Verification items for the finished model (mm, model axes). Round coordinates to 2 decimals unless told otherwise and drop trailing zeros. Write each loop counter-clockwise with the first axis right and the second up, starting at its lowest first coordinate (ties: lowest second). Pieces come first, ordered by that corner, then holes. Notation, with made-up numbers: M 0.25,43 L 30.25,43 A30 ccw 30.25,76 Z; hole C -24.5,-27 d4. An arc over 180 degrees is marked long. Answer in a Markdown table with one row per item. Add a question column.
1. Sectioned sample at C-C on y = -19.5. Record the cut outline in (x, z), plus the area to 3 significant figures.
2. Material ranges on probe 1 along Y at (x, z) = (52, 1563); probe 2 along X at (y, z) = (-2, 1149), recorded low to high.
3. Go/stop test with flat-tipped pins: pin 1 Ø1.5 at (y, z) = (-46.5, 614) entering from -X; pin 2 Ø10 at (y, z) = (-34, 258) entering from +X. Record where each tip stops, or that it passes through.
4. Sectioned sample at A-A on x = -25. Record the cut outline in (y, z), plus the area to 3 significant figures.
5. Sectioned sample at B-B on z = 566.5. Record the cut outline in (x, y), plus the area to 3 significant figures.
```python
from build123d import *

# Parameters (mm, degrees)
BOSS_EXTRUDE1_DEPTH = 2133.6
SKETCH2_W           = 19.05
SKETCH2_H           = 19.05
CUT_EXTRUDE1_DEPTH  = 2136.489044692
FILLET1_R           = 2.54


with BuildPart() as part:
    # Sketch1 → Boss-Extrude1 (new body)
    with BuildSketch(Plane.XY):
        Polygon((-63.5, 63.5), (63.5, 63.5), (63.5, 53.0352), (23.0251, 53.0352), (23.0251, 33.9852), (3.9751, 33.9852), (3.9751, -53.0352), (63.5, -53.0352), (63.5, -63.5), (-63.5, -63.5), (-63.5, -53.0352), (-3.9751, -53.0352), (-3.9751, 33.9852), (-23.0251, 33.9852), (-23.0251, 53.0352), (-63.5, 53.0352), align=None)
    extrude(amount=BOSS_EXTRUDE1_DEPTH)

    # Sketch2 → Cut-Extrude1 (cut, through all)
    with BuildSketch(Plane.XY):
        with Locations((-13.5001, 43.5102)):
            Rectangle(SKETCH2_W, SKETCH2_H)
        with Locations((13.5001, 43.5102)):
            Rectangle(SKETCH2_W, SKETCH2_H)
    extrude(amount=CUT_EXTRUDE1_DEPTH, mode=Mode.SUBTRACT)

    # Fillet1
    fillet1_edges = [part.edges().sort_by_distance(p)[0] for p in [
        (-63.5, -53.0352, 1066.8),
        (-3.9751, -53.0352, 1066.8),
        (-63.5, 53.0352, 1066.8),
        (63.5, 53.0352, 1066.8),
        (3.9751, -53.0352, 1066.8),
        (63.5, -53.0352, 1066.8),
        (-3.9751, 53.0352, 1066.8),
        (3.9751, 53.0352, 1066.8),
    ]]
    fillet(fillet1_edges, radius=FILLET1_R)


solid = part.part
```
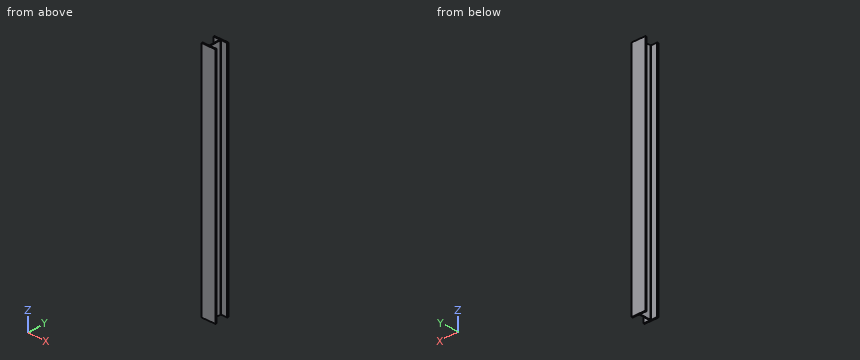
Geometry check:
| question | item | result |
|---|---|---|
| 1 | outline | M -3.98,0 L 3.98,0 L 3.98,2133.6 L -3.98,2133.6 Z |
| 1 | area | 17,000 mm2 |
| 2 | probe 1 | y = -63.5 to -53.04, 53.04 to 63.5 |
| 2 | probe 2 | x = -3.98 to 3.98 |
| 3 | pin 1 | stops at x = -3.98 |
| 3 | pin 2 | stops at x = 3.98 |
| 4 | outline | M -63.5,0 L -53.04,0 L -53.04,2133.6 L -63.5,2133.6 Z; M 53.04,0 L 63.5,0 L 63.5,2133.6 L 53.04,2133.6 Z |
| 4 | area | 44,700 mm2 |
| 5 | outline | M -63.5,-63.5 L 63.5,-63.5 L 63.5,-55.58 A2.54 ccw 60.96,-53.04 L 6.52,-53.04 A2.54 cw 3.98,-50.5 L 3.98,50.5 A2.54 cw 6.52,53.04 L 60.96,53.04 A2.54 ccw 63.5,55.58 L 63.5,63.5 L -63.5,63.5 L -63.5,55.58 A2.54 ccw -60.96,53.04 L -6.52,53.04 A2.54 cw -3.98,50.5 L -3.98,-50.5 A2.54 cw -6.52,-53.04 L -60.96,-53.04 A2.54 ccw -63.5,-55.58 Z |
| 5 | area | 3,500 mm2 |
